Model file for the job. Use its own axes, mm. A direction names the side the tool comes from. Round coordinates to 2 decimals unless told otherwise and drop trailing zeros. Order: outer loops, then holes, each group sorted by start corner. A loop starts at its lowest first (then second) coordinate and runs counter-clockwise, first axis right, second up. Notation, with made-up numbers: (-8, -2.75) -> (14, -2.75) arc R8 ccw to (14, 8.25) -> close; hole circle Ø4 at (21.5, -9.75). An arc over 180 degrees is marked (long way). Answer as CSV lines item,"result".
```python
from build123d import *

# Parameters (mm, degrees)
CHAMFER1_SIZE      = 0.43815
CHAMFER2_SIZE      = 0.232171875
CUT_EXTRUDE2_DEPTH = 1.5875


with BuildPart() as part:
    # Sketch1 → Revolve1 (revolve)
    with BuildSketch(Plane(origin=(0, 0, 0), x_dir=(0, 0, -1), z_dir=(1, 0, 0))):
        Polygon((0, 3.571875), (3.175, 3.571875), (3.175, 1.984375), (19.05, 1.984375), (19.05, 1.7526), (23.8125, 1.7526), (23.8125, 0), (0, 0), align=None)
    revolve(axis=Axis((0, 0, -23.8125), (0, 0, 1)))

    # Sketch5 → Cut-Revolve1 (revolve, cut)
    with BuildSketch(Plane(origin=(0, 0, 0), x_dir=(0, 0, -1), z_dir=(1, 0, 0))):
        with BuildLine():
            Line((19.05, 1.984375), (21.453475, 1.984375))
            Line((21.453475, 1.984375), (20.6502, 1.1811))
            Line((20.6502, 1.1811), (19.6215, 1.1811))
            ThreePointArc((19.6215, 1.1811), (19.217388475, 1.348488475), (19.05, 1.7526))
            Line((19.05, 1.7526), (19.05, 1.984375))
        make_face()
    revolve(axis=Axis((0, 0, -23.8125), (0, 0, 1)), mode=Mode.SUBTRACT)

    # Chamfer1
    chamfer1_edges = [part.edges().sort_by_distance(p)[0] for p in [
        (0, -1.7526, -23.8125),
    ]]
    chamfer(chamfer1_edges, length=CHAMFER1_SIZE)

    # Chamfer2
    chamfer2_edges = [part.edges().sort_by_distance(p)[0] for p in [
        (0, -1.984375, -19.05),
        (0, -3.571875, 0),
    ]]
    chamfer(chamfer2_edges, length=CHAMFER2_SIZE)

    # Sketch8 → Cut-Extrude2 (cut)
    with BuildSketch(Plane.XY):
        Polygon((1.190625, 0.687407664), (0, 1.374815329), (-1.190625, 0.687407664), (-1.190625, -0.687407664), (0, -1.374815329), (1.190625, -0.687407664), align=None)
    extrude(amount=-CUT_EXTRUDE2_DEPTH, mode=Mode.SUBTRACT)

    # Cut-Extrude4 cone 1 section (through the dimple's axis) → Cut-Extrude4 (revolve, cut)
    with BuildSketch(Plane(origin=(0, 0, 0), x_dir=(0, -1, 0), z_dir=(1, 0, 0))):
        Polygon((0, 0), (1.374815329, 0), (0, 1.374815329), align=None)
    revolve(axis=Axis((0, 0, 0), (0, 0, -1)), mode=Mode.SUBTRACT)


solid = part.part
```
Q1. Saw through at B-B (z = -9.75). Write the cut outline in (x, y).
Checks:
outline,"circle Ø3.97 at (0, 0)"
Q2. Tool access for faces 1 (the cylindrical face through (-0.53, 1.67, -22.31)), 2 (the cylindrical face through (-1, 0.63, -20.13)), 3 (the flat face through (-0.6, -1.03, -0.78)): list every direction of +Z, -Z, +X, -X, +Y, -Y with a clear straight run to the whole face (end or side of a thin tool).
Checks:
face 1,"-Z"
face 2,"none"
face 3,"+Z"
Q3. Mould opens along Y. For faces 4 (the cylindrical face through (0.76, 1.833, -11.106)), 5 (the flat face through (0.587, -1.036, -0.783)), 6 (the flat face through (2, 2, -3.175)) say: +Y half, -Y half, draft (parallel to the pull), parting line (faces both ways), or undercut.
Checks:
face 4,"parting line"
face 5,"undercut"
face 6,"draft"
Q4. Flat gauge pins, fed straight in: pin 1 (1.5 mm diameter, centred on y = -2.5, z = -12, fed in from -X); pin 2 (1.9 mm diameter, centred on x = 0, y = 0, fed in from +Z); pin 3 (4 mm diameter, centred on x = 1.5, z = -18.5, fed in from +Y). Where does each tip first touch, or does it go through?
Checks:
pin 1,"x = -0.94"
pin 2,"z = -1.59"
pin 3,"y = 1.98"
Q5. Wall check: L1, parallel to Z at x = -0.5, y = 0.5; L2, parallel to Z at x = 1, y = -0.75; L3, parallel to X at y = 0, z = -6.5. Give the ranges that are in metal, low to high. Write a range as [from, to].
Checks:
L1,"[-23.81, -1.59]"
L2,"[-23.81, -20.72], [-19.35, -1.59]"
L3,"[-1.98, 1.98]"
Q6. Saw through at A-A (z = -22.25). Write the cut outline in (x, y), plus the area to 3 significant figures.
Checks:
outline,"circle Ø3.51 at (0, 0)"
area,"9.65 mm²"
